Work out the finished part from the listing and answer in its coordinate system (mm). Face numbers are marked on the shaded views. A direction names the side the tool comes from. Give positions to 0.01 mm unless a question says otherwise; leave off trailing zeros. Order: outer loops, then holes, each group sorted by start corner. A loop starts at its lowest first (then second) coordinate and runs counter-clockwise, first axis right, second up. Notation, with made-up numbers: (33.25, 82) - (74.25, 82) arc R9 ccw to (74.25, 98) - close; hole circle Ø8 at (85, -40). An arc over 180 degrees is marked (long way). Put each result on its own line as item: value.
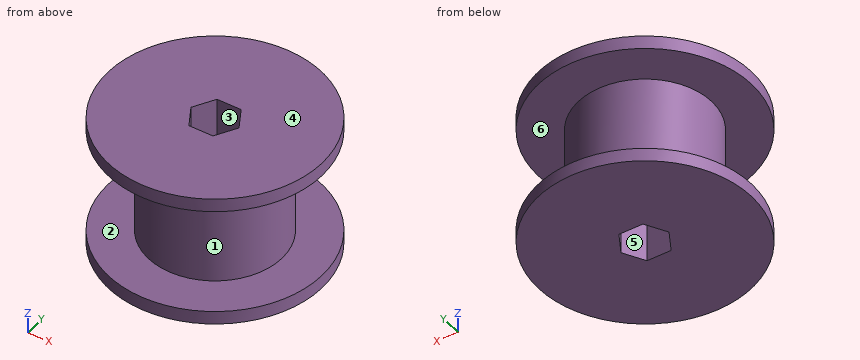
```python
from build123d import *

# Parameters (mm, degrees)
SKETCH1_R        = 15.875
DRUM_DEPTH       = 12.7
SKETCH3_R        = 25.4
FLANGE_DEPTH     = 3.175
ATTACHMENT_DEPTH = 48.941448664


with BuildPart() as part:
    # Sketch1 → Drum (new, symmetric)
    with BuildSketch(Plane.XY):
        Circle(SKETCH1_R)
    extrude(amount=DRUM_DEPTH, both=True)

    # Sketch3 → Flange (add)
    with BuildSketch(Plane.XY.offset(12.7)):
        Circle(SKETCH3_R)
    flange = extrude(amount=FLANGE_DEPTH)

    # Flange2: Flange across plane
    add(flange.mirror(Plane.XY))

    # Sketch4 → Attachment (cut, through all)
    with BuildSketch(Plane.XY.offset(15.875)):
        Polygon((5.719231767, 0), (2.859615883, 4.953), (-2.859615883, 4.953), (-5.719231767, 0), (-2.859615883, -4.953), (2.859615883, -4.953), align=None)
    extrude(amount=-ATTACHMENT_DEPTH, mode=Mode.SUBTRACT)


solid = part.part
```
(1) A tool of negligible diameter and unlimited length cuts with its end or side. For the marked faces 4, 5 and 6, from which of +Z, -Z, +X, -X, +Y, -Y can it reach the whole face along a straight path? Write none if from no direction.
Geometry check:
face 4: +Z, +X, -X, +Y, -Y
face 5: +Z, -Z
face 6: none
(2) Given pin 1 (4 mm diameter, centred on y = -15, z = -2.5, fed in from -X); pin 2 (6 mm diameter, centred on x = -4, z = -1.5, fed in from +Y); pin 3 (5 mm diameter, centred on x = 10.5, z = 3.5, fed in from -Y), each flat-ended and moving along its own axis, determine where each tip first touches the part or whether it passes through.
Geometry check:
pin 1: stops at x = -9.11
pin 2: stops at y = 15.84
pin 3: stops at y = -13.71
(3) Section A-A, the plane z = -10.5 is taken. Write down the section's boundary in (x, y) (3 decimals), then the cut area to 3 significant figures.
Geometry check:
outline: circle Ø31.75 at (0, 0); hole (-5.719, 0) - (-2.86, -4.953) - (2.86, -4.953) - (5.719, 0) - (2.86, 4.953) - (-2.86, 4.953) - close
area: 707 mm²
(4) Straight lines are drawn through the part: line 1 (Z direction, x = -1.5, y = 23.5) (3 decimals); line 2 (Y direction, x = -0.5, z = 0.5); line 3 (Y direction, x = 3.5, z = 9). For each, find the intervals that lie inside material, in ascending order.
Geometry check:
line 1: z = -15.875 to -12.7, 12.7 to 15.875
line 2: y = -15.87 to -4.95, 4.95 to 15.87
line 3: y = -15.48 to -3.84, 3.84 to 15.48
(5) Section C-C, the plane y = 19 is taken. Write down the section's boundary in (x, z) (3 decimals), then the cut area to 3 significant figures.
Geometry check:
outline: (-16.857, -15.875) - (16.857, -15.875) - (16.857, -12.7) - (-16.857, -12.7) - close; (-16.857, 12.7) - (16.857, 12.7) - (16.857, 15.875) - (-16.857, 15.875) - close
area: 214 mm²
(6) Section D-D, the plane y = -11.5 is taken. Write down the section's boundary in (x, z) (3 decimals), then the cut area to 3 significant figures.
Geometry check:
outline: (-22.648, -15.875) - (22.648, -15.875) - (22.648, -12.7) - (10.944, -12.7) - (10.944, 12.7) - (22.648, 12.7) - (22.648, 15.875) - (-22.648, 15.875) - (-22.648, 12.7) - (-10.944, 12.7) - (-10.944, -12.7) - (-22.648, -12.7) - close
area: 844 mm²
(7) Determine the mould class of the marked faces 1, 2 and 3 for opening direction X: pulls with the +X half, pulls with the -X half, needs draft (parallel to the pull), parting line crosses it, or undercut.
Geometry check:
face 1: parting line crosses it
face 2: needs draft
face 3: undercut
(8) Section B-B, the plane x = 0 is taken. Write down the section's boundary in (y, z) (3 decimals).
Geometry check:
outline: (-25.4, -15.875) - (-4.953, -15.875) - (-4.953, 15.875) - (-25.4, 15.875) - (-25.4, 12.7) - (-15.875, 12.7) - (-15.875, -12.7) - (-25.4, -12.7) - close; (4.953, -15.875) - (25.4, -15.875) - (25.4, -12.7) - (15.875, -12.7) - (15.875, 12.7) - (25.4, 12.7) - (25.4, 15.875) - (4.953, 15.875) - close
